Check sheet for the modelled part. Datum: model origin and axes. Units: mm. A direction names the side the tool comes from. Round coordinates to 2 decimals unless told otherwise and drop trailing zeros. Order: outer loops, then holes, each group sorted by start corner. A loop starts at its lowest first (then second) coordinate and runs counter-clockwise, first axis right, second up. Notation, with made-up numbers: (3.5, 18) -> (61.5, 18) arc R9 ccw to (61.5, 26) -> close; hole circle Ø7 at (-1.75, -1). An arc over 180 degrees is marked (long way). Answer in a Markdown table with one row per item. Add a question column.
1. Sectioned sample at B-B, the plane y = 1.75. Record the boundary of the cut face in (x, z).
2. Sectioned sample at C-C, the plane z = 0. Record the boundary of the cut face in (x, y), then the cut area to 3 significant figures.
3. Draft check along X on faces 4 (the flat face through (-200, 5, 0)), 5 (the flat face through (114, 5, 25)), 6 (the cylindrical face through (9.76, 3.45, -31)). Enter one of: +X half, -X half, draft (parallel to the pull), parting line (faces both ways), or undercut.
4. Material ranges on L1, parallel to X at y = 3, z = 0; L2, parallel to Z at x = 159, y = 3; L3, parallel to X at y = 8.4, z = 0, recorded low to high. Write a range as from..to.
5. Sectioned sample at A-A, the plane x = 0. Record the boundary of the cut face in (y, z), then the cut area to 3 significant figures.
6. Access from +Z, -Z, +X, -X, +Y, -Y to the whole of each face (thin tool, end or side, straight path). Record for faces 1 (the flat face through (-114, 5, -25)), 2 (the flat face through (117, 5, -25)), 3 (the flat face through (-117, 5, 25)).
7. Sectioned sample at D-D, the plane x = -156. Record the boundary of the cut face in (y, z), then the cut area to 3 significant figures.
8. Depth check by flat-ended pin: P1, Ø5, axis at x = 111, y = 2.5, coming from the -Z side; P2, Ø5, axis at x = 117.5, y = 7, coming from the +Z side. Enter the tip coordinate at first touch or a pass-through.
```python
from build123d import *

# Parameters (mm, degrees)
BOSS_EXTRUDE1_DEPTH = 10
CUT_EXTRUDE3_REACH  = 206.206
SKETCH4_R           = 30.5
SKETCH3_R           = 32.5
CUT_EXTRUDE4_DEPTH  = 7


with BuildPart() as part:
    # Sketch1 → Boss-Extrude1 (new body)
    with BuildSketch(Plane(origin=(0, 0, 0), x_dir=(1, 0, 0), z_dir=(0, 1, 0))):
        with BuildLine():
            ThreePointArc((31.224989992, 25), (0, 40), (-31.224989992, 25))
            Line((-31.224989992, 25), (31.224989992, 25))
        make_face()
        with BuildLine():
            Line((31.224989992, 25), (-31.224989992, 25))
            ThreePointArc((-31.224989992, 25), (-40, 0), (-31.224989992, -25))
            Line((-31.224989992, -25), (31.224989992, -25))
            ThreePointArc((31.224989992, -25), (37.742546282, -13.247648854), (40, 0))
            ThreePointArc((40, 0), (37.742546282, 13.247648854), (31.224989992, 25))
        make_face()
        with BuildLine():
            Line((-31.224989992, 25), (-200, 25))
            Line((-200, 25), (-200, -25))
            Line((-200, -25), (-31.224989992, -25))
            ThreePointArc((-31.224989992, -25), (-40, 0), (-31.224989992, 25))
        make_face()
        with BuildLine():
            Line((200, 25), (31.224989992, 25))
            ThreePointArc((31.224989992, 25), (37.742546282, 13.247648854), (40, 0))
            ThreePointArc((40, 0), (37.742546282, -13.247648854), (31.224989992, -25))
            Line((31.224989992, -25), (200, -25))
            Line((200, -25), (200, 25))
        make_face()
        with BuildLine():
            Line((31.224989992, -25), (-31.224989992, -25))
            ThreePointArc((-31.224989992, -25), (0, -40), (31.224989992, -25))
        make_face()
    extrude(amount=BOSS_EXTRUDE1_DEPTH)

    # Sketch4 → Cut-Extrude3 (cut, up to next)
    with BuildSketch(Plane(origin=(0, 10, 0), x_dir=(1, 0, 0), z_dir=(0, 1, 0)), mode=Mode.PRIVATE) as cut_extrude3_sk1:
        with Locations(Location((0, 0, 0), (0, 0, 270))):
            Circle(SKETCH4_R)
    cut_extrude3_tool1 = extrude(cut_extrude3_sk1.sketch, amount=-CUT_EXTRUDE3_REACH, mode=Mode.PRIVATE) & part.part
    add(cut_extrude3_tool1.solids().sort_by_distance((0, 10, 0))[0], mode=Mode.SUBTRACT)

    # Sketch3 → Cut-Extrude4 (cut)
    with BuildSketch(Plane.XZ):
        with Locations(Location((0, 0, 0), (0, 0, 270))):
            Circle(SKETCH3_R)
    extrude(amount=-CUT_EXTRUDE4_DEPTH, mode=Mode.SUBTRACT)


solid = part.part
```
Answer key:
| question | item | result |
|---|---|---|
| 1 | outline | (-200, -25) -> (-31.22, -25) arc R40 ccw to (31.22, -25) -> (200, -25) -> (200, 25) -> (31.22, 25) arc R40 ccw to (-31.22, 25) -> (-200, 25) -> close; hole circle Ø65 at (0, 0) |
| 2 | outline | (-200, 0) -> (-32.5, 0) -> (-32.5, 7) -> (-30.5, 7) -> (-30.5, 10) -> (-200, 10) -> close; (30.5, 7) -> (32.5, 7) -> (32.5, 0) -> (200, 0) -> (200, 10) -> (30.5, 10) -> close |
| 2 | area | 3,360 mm² |
| 3 | face 4 | -X half |
| 3 | face 5 | draft |
| 3 | face 6 | undercut |
| 4 | L1 | x = -200..-32.5, 32.5..200 |
| 4 | L2 | z = -25..25 |
| 4 | L3 | x = -200..-30.5, 30.5..200 |
| 5 | outline | (0, -40) -> (10, -40) -> (10, -30.5) -> (7, -30.5) -> (7, -32.5) -> (0, -32.5) -> close; (0, 32.5) -> (7, 32.5) -> (7, 30.5) -> (10, 30.5) -> (10, 40) -> (0, 40) -> close |
| 5 | area | 162 mm² |
| 6 | face 1 | -Z, -X, +Y, -Y |
| 6 | face 2 | -Z, +X, +Y, -Y |
| 6 | face 3 | +Z, -X, +Y, -Y |
| 7 | outline | (0, -25) -> (10, -25) -> (10, 25) -> (0, 25) -> close |
| 7 | area | 500 mm² |
| 8 | P1 | stops at z = -25 |
| 8 | P2 | stops at z = 25 |
